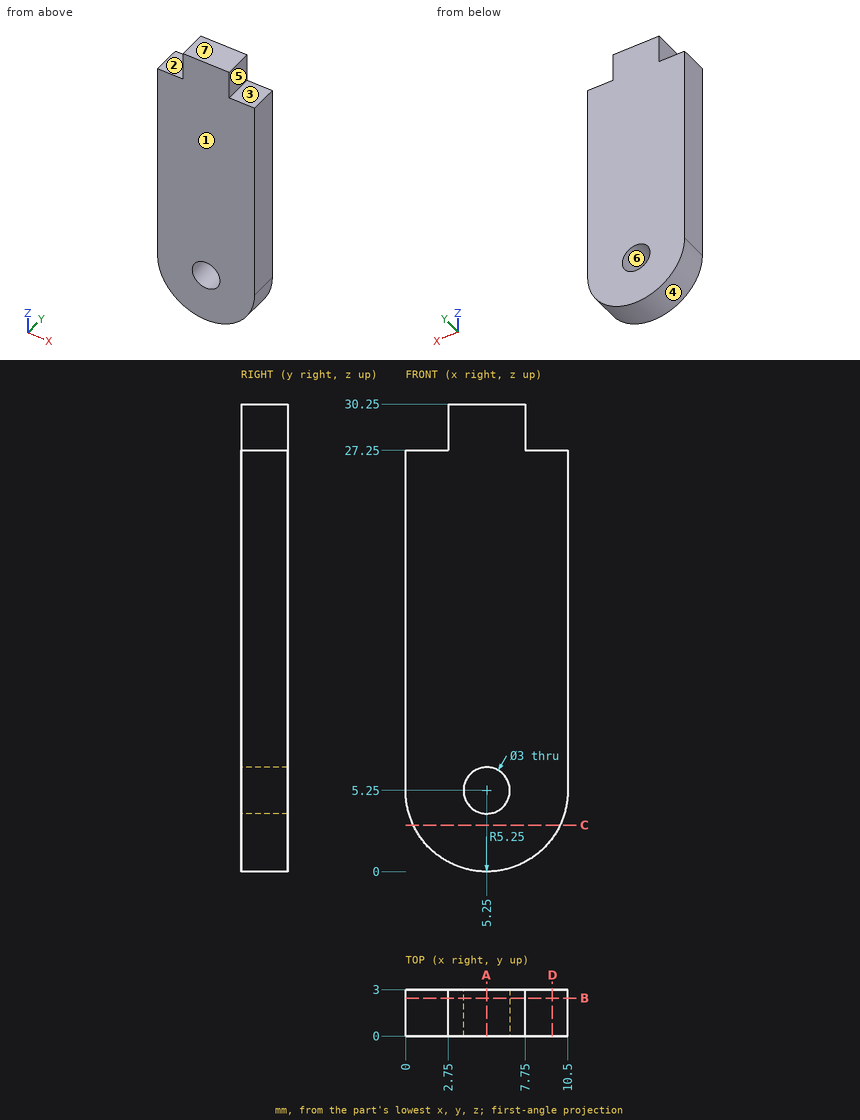
Verification items for this drawing (mm, ordinates from the low corner). A direction names the side the tool comes from. Coordinates: 2 decimals unless noted, no trailing zeros. Order: outer loops, then holes, each group sorted by start corner. A loop starts at its lowest first (then second) coordinate and runs counter-clockwise, first axis right, second up. Notation, with made-up numbers: (67, -12) - (90, -12) arc R14 ccw to (90, 9) - close; hole circle Ø6 at (10, 5). An arc over 180 degrees is marked (long way). Use one line per item in the form item = value.
1. Section check B-B (y = 2.45). Record the boundary of the cut face in (x, z).
Here are the results:
outline = (0, 5.25) arc R5.25 ccw to (10.5, 5.25) - (10.5, 27.25) - (7.75, 27.25) - (7.75, 30.25) - (2.75, 30.25) - (2.75, 27.25) - (0, 27.25) - close; hole circle Ø3 at (5.25, 5.25)
2. Section check D-D (x = 9.5). Record the boundary of the cut face in (y, z).
Here are the results:
outline = (0, 2.17) - (3, 2.17) - (3, 27.25) - (0, 27.25) - close
3. Section check A-A (x = 5.25). Record the boundary of the cut face in (y, z), then the cut area to 4 significant figures.
Here are the results:
outline = (0, 0) - (3, 0) - (3, 3.75) - (0, 3.75) - close; (0, 6.75) - (3, 6.75) - (3, 30.25) - (0, 30.25) - close
area = 81.75 mm²
4. Scan lines: line 1 (Z direction, x = 5.25, y = 1.3); line 2 (X direction, y = 0.85, z = 5.25); line 3 (X direction, y = 1.9, z = 4). Record each from-to range of solid material in increasing order.
Here are the results:
line_1 = 0 to 3.75, 6.75 to 30.25
line_2 = 0 to 3.75, 6.75 to 10.5
line_3 = 0.15 to 4.42, 6.08 to 10.35
5. Access from +Z, -Z, +X, -X, +Y, -Y to the whole of each face (thin tool, end or side, straight path). Record for the marked faces 1, 2 and 3.
Here are the results:
face_1 = +Z, -Z, +X, -X, -Y
face_2 = +Z, -X, +Y, -Y
face_3 = +Z, +X, +Y, -Y
6. Draft check along Z on the marked faces 4, 5, 6 and 7. Enter one of: pulls with the +Z half, pulls with the -Z half, needs draft (parallel to the pull), parting line crosses it, or undercut.
Here are the results:
face_4 = pulls with the -Z half
face_5 = needs draft
face_6 = undercut
face_7 = pulls with the +Z half
7. Section check C-C (z = 3). Record the boundary of the cut face in (x, y), then the cut area to 3 significant figures.
Here are the results:
outline = (0.51, 0) - (9.99, 0) - (9.99, 3) - (0.51, 3) - close
area = 28.5 mm²
8. Gauge pin test, flat ends, axial feed: pin 1 (0.9 mm diameter, centred on y = 1.5, z = 29, fed in from +X); pin 2 (1 mm diameter, centred on y = 2, z = 4, fed in from -X); pin 3 (2.5 mm diameter, centred on x = 5.25, z = 5.25, fed in from -Y). Record the tip position at first contact, or that the pin passes through.
Here are the results:
pin_1 = 7.75
pin_2 = 0.05
pin_3 = through
